The drawing under review shows one solid part. Ordinate dimensions are in mm from its lowest x, y, z. Give positions to 0.01 mm unless a question says otherwise; leave off trailing zeros. Loops run counter-clockwise (first coordinate to the right, second up) from the corner with the lowest first, then second, coordinate; pieces in that order, holes last.
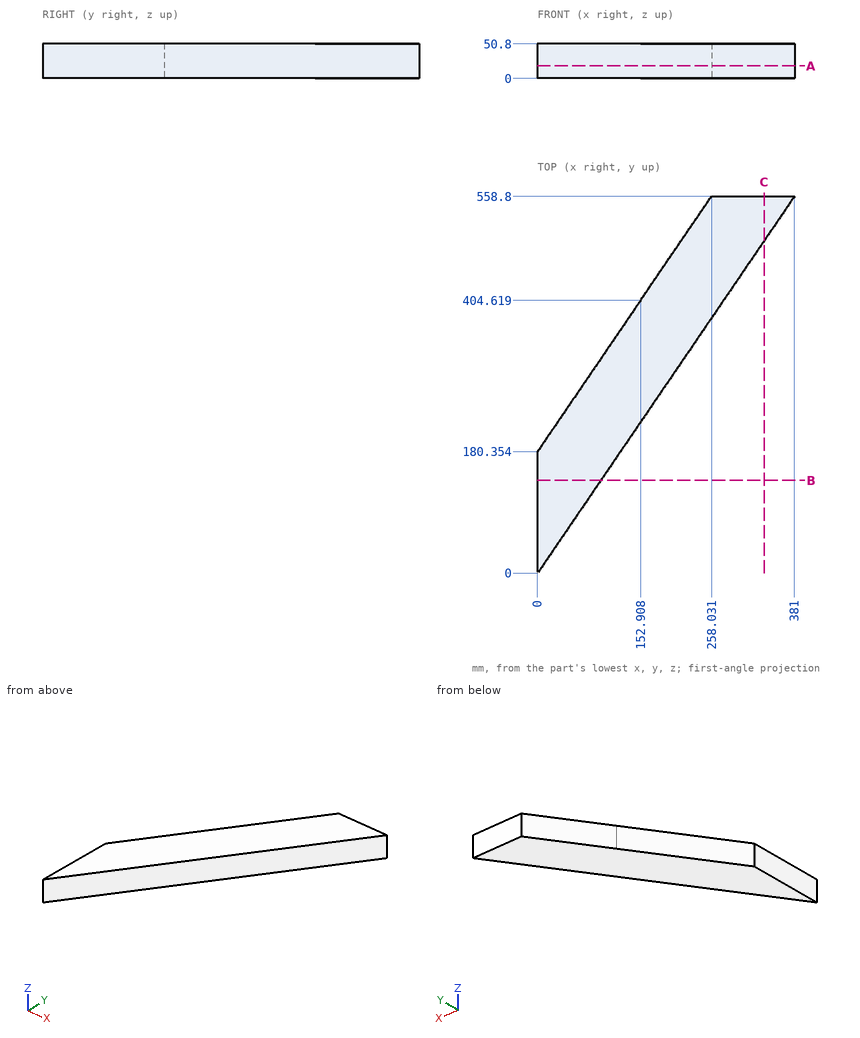
Item 1: Clearance check with flat-ended pins moving along their axes: pin 1 Ø10 at (y, z) = (480, 43) entering from -X (1 decimal); pin 2 Ø4 at (x, z) = (342, 45.5) entering from -Y (1 decimal); pin 3 Ø8 at (x, y) = (70.5, 291.5) entering from -Z; pin 4 Ø2 at (y, z) = (450, 17) entering from +X. State where each tip first meets the part, or that it passes through.
Answer:
pin 1: stops at x = 200.9
pin 2: stops at y = 498.7
pin 3: passes through
pin 4: stops at x = 307.5
Item 2: For L1, parallel to X at y = 379, z = 19; L2, parallel to X at y = 376.5, z = 34.5 (1 decimal); L3, parallel to Y at x = 357, z = 21, list the stretches that pass through material, from the lowest coordinate up.
Answer:
L1: x = 135.44 to 258.41
L2: x = 133.7 to 256.7
L3: y = 523.6 to 558.8
Item 3: Take a section at B-B on y = 137.5. Give the boundary of the cut face in (x, z), and give its area (3 significant figures).
Answer:
outline: (0, 0) - (93.75, 0) - (93.75, 50.8) - (0, 50.8) - close
area: 4,760 mm2
Item 4: Take a section at A-A on z = 18.5. Give the boundary of the cut face in (x, y).
Answer:
outline: (0, 0) - (381, 558.8) - (258.03, 558.8) - (152.91, 404.62) - (0, 180.35) - close
Item 5: Take a section at C-C on x = 336. Give the boundary of the cut face in (y, z), and give its area (3 significant figures).
Answer:
outline: (492.8, 0) - (558.8, 0) - (558.8, 50.8) - (492.8, 50.8) - close
area: 3,350 mm2
